Can you work these out from the model? Positions are in its coordinate system, mm. A direction names the side the tool comes from. Give positions to 0.01 mm unless a question says otherwise; leave off trailing zeros. Loops run counter-clockwise (first coordinate to the right, second up) from the corner with the lowest first, then second, coordinate; pieces in that order, holes last.
from build123d import *

# Parameters (mm, degrees)
F0_W     = 63.5
F0_H     = 101.6
F1_DEPTH = 9.525
F2_T     = -2.54
F3_R     = 1.016


with BuildPart() as f1:
    # F0 (on Top) → F1 (new body)
    with BuildSketch(Plane.XY):
        Rectangle(F0_W, F0_H)
    extrude(amount=F1_DEPTH)

    # F2
    f2_openings = [f1.faces().sort_by_distance(p)[0] for p in [
        (0, 0, 9.525),
    ]]
    offset(amount=F2_T, openings=f2_openings)

    # F3
    f3_edges = [f1.edges().sort_by_distance(p)[0] for p in [
        (-31.75, 0, 0),
        (0, -50.8, 0),
        (31.75, 0, 0),
        (0, 50.8, 0),
        (-31.75, 0, 9.525),
        (0, -50.8, 9.525),
        (31.75, 0, 9.525),
        (0, 50.8, 9.525),
        (-29.21, 0, 9.525),
        (0, 48.26, 9.525),
        (29.21, 0, 9.525),
        (0, -48.26, 9.525),
        (-31.75, 50.8, 4.7625),
        (-31.75, -50.8, 4.7625),
        (31.75, 50.8, 4.7625),
        (31.75, -50.8, 4.7625),
    ]]
    fillet(f3_edges, radius=F3_R)


solid = f1.part
(1) Which directions (+Z, -Z, +X, -X, +Y, -Y) give clear straight access to the entire face, cutting with the end or side of a thin tool? Please do faces 1 (the flat face through (31.75, -1, 5)), 2 (the flat face through (0, 1, 2.54)).
Returned:
face 1: +Z, -Z, +X, +Y, -Y
face 2: +Z
(2) Suppose I cut it at A-A on z = 7.25. List the corners of the cut face in (x, y) for me, plus the area to 3 significant figures.
Returned:
outline: (-31.75, -49.78) arc R1.02 ccw to (-30.73, -50.8) - (30.73, -50.8) arc R1.02 ccw to (31.75, -49.78) - (31.75, 49.78) arc R1.02 ccw to (30.73, 50.8) - (-30.73, 50.8) arc R1.02 ccw to (-31.75, 49.78) - close; hole (-29.21, -48.26) - (29.21, -48.26) - (29.21, 48.26) - (-29.21, 48.26) - close
area: 812 mm2
(3) Thinking about a two-plate mould opening in X: for faces 3 (the flat face through (0, 50.8, 5)), 4 (the flat face through (-31.75, -1, 5)), 5 (the flat face through (29.21, -1, 5)), 6 (the flat face through (0, -48.26, 5)), which applies, pulls with the +X half, pulls with the -X half, needs draft (parallel to the pull), parting line crosses it, or undercut?
Returned:
face 3: needs draft
face 4: pulls with the -X half
face 5: undercut
face 6: undercut
(4) Will this pin go through, and if not, where does the flat tip stop? P1, Ø3, axis at x = -2, y = 35.5, coming from the +Z side.
Returned:
P1: stops at z = 2.54
(5) Suppose I cut it at B-B on y = 34. List the corners of the cut face in (x, z) for me (3 decimals).
Returned:
outline: (-31.75, 1.016) arc R1.016 ccw to (-30.734, 0) - (30.734, 0) arc R1.016 ccw to (31.75, 1.016) - (31.75, 8.509) arc R1.016 ccw to (30.734, 9.525) - (30.226, 9.525) arc R1.016 ccw to (29.21, 8.509) - (29.21, 2.54) - (-29.21, 2.54) - (-29.21, 8.509) arc R1.016 ccw to (-30.226, 9.525) - (-30.734, 9.525) arc R1.016 ccw to (-31.75, 8.509) - close
(6) Please list where these lines run through material, in increasing order: probe 1 along X at (y, z) = (-16, 4.5); probe 2 along Y at (x, z) = (-28, 7.25); probe 3 along Z at (x, y) = (-3, 12).
Returned:
probe 1: x = -31.75 to -29.21, 29.21 to 31.75
probe 2: y = -50.8 to -48.26, 48.26 to 50.8
probe 3: z = 0 to 2.54
(7) Suppose I cut it at C-C on x = 11. List the corners of the cut face in (y, z) for me (3 decimals).
Returned:
outline: (-50.8, 1.016) arc R1.016 ccw to (-49.784, 0) - (49.784, 0) arc R1.016 ccw to (50.8, 1.016) - (50.8, 8.509) arc R1.016 ccw to (49.784, 9.525) - (49.276, 9.525) arc R1.016 ccw to (48.26, 8.509) - (48.26, 2.54) - (-48.26, 2.54) - (-48.26, 8.509) arc R1.016 ccw to (-49.276, 9.525) - (-49.784, 9.525) arc R1.016 ccw to (-50.8, 8.509) - close
